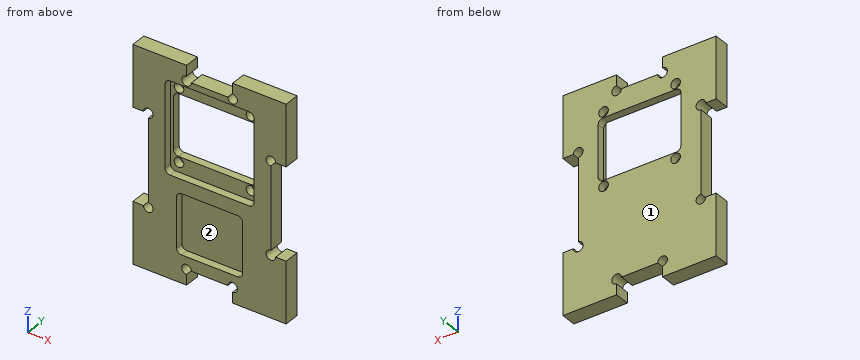
```python
from build123d import *

# Parameters (mm, degrees)
SKETCH1_W               = 50
SKETCH1_H               = 70
BOSS_EXTRUDE1_DEPTH     = 5
CUT_EXTRUDE1_DEPTH      = 2.5
SKETCH3_R               = 1.57480315
CUT_EXTRUDE5_DEPTH      = 6
CUT_EXTRUDE2_DEPTH      = 2.5
SKETCH5_W               = 5
SKETCH5_H               = 30
SKETCH5_W_2             = 15
SKETCH5_H_2             = 5
CUT_EXTRUDE3_DEPTH      = 1
CUT_EXTRUDE3_DEPTH_BACK = 6
SKETCH6_R               = 1.57480315
CUT_EXTRUDE4_DEPTH      = 6


with BuildPart() as part:
    # Sketch1 → Boss-Extrude1 (new body)
    with BuildSketch(Plane(origin=(0, 0, 0), x_dir=(1, 0, 0), z_dir=(0, 1, 0))):
        with Locations((25, 35)):
            Rectangle(SKETCH1_W, SKETCH1_H)
        with BuildLine():
            Line((13.07480315, 12), (36.92519685, 12))
            ThreePointArc((36.92519685, 12), (38.038750837, 12.461249163), (38.5, 13.57480315))
            Line((38.5, 13.57480315), (38.5, 30.42519685))
            ThreePointArc((38.5, 30.42519685), (38.038750837, 31.538750837), (36.92519685, 32))
            Line((36.92519685, 32), (13.07480315, 32))
            ThreePointArc((13.07480315, 32), (11.961249163, 31.538750837), (11.5, 30.42519685))
            Line((11.5, 30.42519685), (11.5, 13.57480315))
            ThreePointArc((11.5, 13.57480315), (11.961249163, 12.461249163), (13.07480315, 12))
        make_face(mode=Mode.SUBTRACT)
    extrude(amount=BOSS_EXTRUDE1_DEPTH)

    # Sketch2 → Cut-Extrude1 (cut)
    with BuildSketch(Plane.XZ):
        with BuildLine():
            Line((12.07480315, -37), (37.92519685, -37))
            ThreePointArc((37.92519685, -37), (39.038750837, -36.538750837), (39.5, -35.42519685))
            Line((39.5, -35.42519685), (39.5, -8.57480315))
            ThreePointArc((39.5, -8.57480315), (39.038750837, -7.461249163), (37.92519685, -7))
            Line((37.92519685, -7), (12.07480315, -7))
            ThreePointArc((12.07480315, -7), (10.961249163, -7.461249163), (10.5, -8.57480315))
            Line((10.5, -8.57480315), (10.5, -35.42519685))
            ThreePointArc((10.5, -35.42519685), (10.961249163, -36.538750837), (12.07480315, -37))
        make_face()
    extrude(amount=-CUT_EXTRUDE1_DEPTH, mode=Mode.SUBTRACT)

    # Sketch3 → Cut-Extrude5 (cut, through all)
    with BuildSketch(Plane(origin=(0, 5, 0), x_dir=(1, 0, 0), z_dir=(0, 1, 0))):
        with Locations((13.25, 33.875)):
            Circle(SKETCH3_R)
        with Locations((36.75, 33.875)):
            Circle(SKETCH3_R)
        with Locations((36.75, 10.125)):
            Circle(SKETCH3_R)
        with Locations((13.25, 10.125)):
            Circle(SKETCH3_R)
    extrude(amount=-CUT_EXTRUDE5_DEPTH, mode=Mode.SUBTRACT)

    # Sketch4 → Cut-Extrude2 (cut)
    with BuildSketch(Plane.XZ):
        with BuildLine():
            Line((34.17519685, -61), (15.82480315, -61))
            ThreePointArc((15.82480315, -61), (14.711249163, -60.538750837), (14.25, -59.42519685))
            Line((14.25, -59.42519685), (14.25, -43.07480315))
            ThreePointArc((14.25, -43.07480315), (14.711249163, -41.961249163), (15.82480315, -41.5))
            Line((15.82480315, -41.5), (34.17519685, -41.5))
            ThreePointArc((34.17519685, -41.5), (35.288750837, -41.961249163), (35.75, -43.07480315))
            Line((35.75, -43.07480315), (35.75, -59.42519685))
            ThreePointArc((35.75, -59.42519685), (35.288750837, -60.538750837), (34.17519685, -61))
        make_face()
    extrude(amount=-CUT_EXTRUDE2_DEPTH, mode=Mode.SUBTRACT)

    # Sketch5 → Cut-Extrude3 (cut, two sides)
    with BuildSketch(Plane(origin=(0, 5, 0), x_dir=(1, 0, 0), z_dir=(0, 1, 0))) as cut_extrude3_sk:
        with Locations((2.5, 35)):
            Rectangle(SKETCH5_W, SKETCH5_H)
        with Locations((25, 67.5)):
            Rectangle(SKETCH5_W_2, SKETCH5_H_2)
        with Locations((47.5, 35)):
            Rectangle(SKETCH5_W, SKETCH5_H)
        with Locations((25, 2.5)):
            Rectangle(SKETCH5_W_2, SKETCH5_H_2)
    extrude(amount=CUT_EXTRUDE3_DEPTH, mode=Mode.SUBTRACT)
    extrude(cut_extrude3_sk.sketch, amount=-CUT_EXTRUDE3_DEPTH_BACK, mode=Mode.SUBTRACT)

    # Sketch6 → Cut-Extrude4 (cut, through all)
    with BuildSketch(Plane.XZ):
        with Locations((5, -50)):
            Circle(SKETCH6_R)
        with Locations((5, -20)):
            Circle(SKETCH6_R)
        with Locations((17.5, -5)):
            Circle(SKETCH6_R)
        with Locations((32.5, -5)):
            Circle(SKETCH6_R)
        with Locations((45, -20)):
            Circle(SKETCH6_R)
        with Locations((45, -50)):
            Circle(SKETCH6_R)
        with Locations((32.5, -65)):
            Circle(SKETCH6_R)
        with Locations((17.5, -65)):
            Circle(SKETCH6_R)
    extrude(amount=-CUT_EXTRUDE4_DEPTH, mode=Mode.SUBTRACT)


solid = part.part
```
Check sheet for the modelled part. Datum: model origin and axes. Units: mm. Face numbers are marked on the shaded views. Coordinates: 2 decimals unless noted, no trailing zeros. Write each loop counter-clockwise with the first axis right and the second up, starting at its lowest first coordinate (ties: lowest second). Pieces come first, ordered by that corner, then holes. Notation, with made-up numbers: (65, 24.5) - (112, 24.5) arc R32 cw to (112, 56.5) - close; hole circle Ø11 at (52, 41.25). An arc over 180 degrees is marked (long way). One line per question, with ' | ' between items.
Item 1: Mould release check, pull along X, two halves, no side actions. Record for the marked faces 1 and 2: pulls with the +X half, pulls with the -X half, needs draft (parallel to the pull), parting line crosses it, or undercut.
Determined:
face 1: needs draft | face 2: undercut
Item 2: Sectioned sample at A-A on x = 27.5. Record the boundary of the cut face in (y, z).
Determined:
outline: (0, -65) - (5, -65) - (5, -32) - (2.5, -32) - (2.5, -37) - (0, -37) - (0, -41.5) - (2.5, -41.5) - (2.5, -61) - (0, -61) - close; (0, -7) - (2.5, -7) - (2.5, -12) - (5, -12) - (5, -5) - (0, -5) - close
Item 3: Gauge pin test, flat ends, axial feed: P1, Ø4, axis at x = 13.25, z = -10.125, coming from the -Y side; P2, Ø2, axis at x = 28, y = 1.5, coming from the -Z side; P3, Ø3, axis at y = 1.5, z = -27, coming from the -X side; P4, Ø2.5, axis at x = 13.25, z = -33.875, coming from the +Y side. Record the tip position at first contact, or that the pin passes through.
Determined:
P1: stops at y = 2.5 | P2: stops at z = -65 | P3: stops at x = 5 | P4: passes through
Item 4: Thickness scan on line 1 (Z direction, x = 26, y = 0.55); line 2 (Z direction, x = 3, y = 1.8); line 3 (X direction, y = 3.4, z = -64). Record the ranges inside material, lowest first. Write a range as [from, to].
Determined:
line 1: z = [-65, -61], [-41.5, -37], [-7, -5] | line 2: z = [-70, -50], [-20, 0] | line 3: x = [0, 16.28], [18.72, 31.28], [33.72, 50]
Item 5: Sectioned sample at B-B on y = 4.05. Give the number of separate pieces and of enclosed holes in the cut face, plus the area to 3 significant figures.
Determined:
separate pieces: 1 | enclosed holes: 5 | area: 2,430 mm2
